Verification items for the finished model (mm, model axes). A direction names the side the tool comes from. Give positions to 0.01 mm unless a question says otherwise; leave off trailing zeros. Order: outer loops, then holes, each group sorted by start corner. A loop starts at its lowest first (then second) coordinate and runs counter-clockwise, first axis right, second up. Notation, with made-up numbers: (57.5, 9) -> (71.5, 9) arc R17 ccw to (71.5, 15) -> close; hole circle Ø3 at (10, -10). An arc over 180 degrees is marked (long way). Return JSON: item names as keys, results as strings. Group by question number.
(1) Cross-section at C-C on x = -0.5. Enter the section's corners in (y, z).
(2) Tool access check on faces 1 (the face through (13.646, 13.93, 0.592)), 2 (the face through (-18.697, -18.759, 3.566)), 3 (the face through (19.359, 19.297, 3.972)). Record the directions out of +Z, -Z, +X, -X, +Y, -Y that give a thin tool (end or side, any length) a straight path to the whole face; none if there is none.
(3) Cross-section at D-D on x = -12.5. Enter the section's corners in (y, z), then the cut area to 3 significant figures.
(4) Release check for a two-part mould opening along X. For faces 4 (the face through (-19.297, 19.359, 3.972)), 5 (the face through (1, -13, 1)), 6 (the face through (20.5, 0, 4)) record: pulls with the +X half, pulls with the -X half, needs draft (parallel to the pull), parting line crosses it, or undercut.
(5) Thickness scan on line 1 along Y through (x, z) = (14, 2.5); line 2 along X through (y, z) = (8, 5); line 3 along Z through (x, y) = (11.5, 3). Record the ranges inside material, lowest first.
(6) Cross-section at A-A on z = 4. Enter the section's corners in (x, y), then the cut area to 4 significant figures.
(7) Cross-section at B-B on y = -13. Enter the section's corners in (x, z).
(8) Depth check by flat-ended pin: pin 1 Ø3 at (x, y) = (12.5, 3) entering from +Z; pin 2 Ø1 at (x, z) = (-8.5, 0.5) entering from +Y; pin 3 Ø1.3 at (y, z) = (-9, 0.5) entering from -X; pin 4 Ø3 at (x, y) = (15.9, 15.9) entering from -Z. Enter the tip coordinate at first touch or a pass-through.
from build123d import *

# Parameters (mm, degrees)
F0_R         = 1.75
F1_DEPTH     = 1.2
F2_DEPTH     = 6
F4_DEPTH     = 10
F5_T1_DEPTH  = 33
F5_T3_DEPTH  = 33
F5_T6_ANGLE  = 90
F5_T8_ANGLE  = 90
F5_T10_ANGLE = 90
F5_T12_ANGLE = 90
F6_DEPTH     = 0.1
F7_DEPTH     = 0.1
F8_DEPTH     = 0.1


# Not quite as in the source:
# - a fillet or chamfer that OpenCascade refuses, or shapes differently, is made with other operations: its cross-section is extruded or revolved along the edge and cut away or added


with BuildPart() as f1:
    # F0 (on Top) → F1 (new body)
    with BuildSketch(Plane.XY):
        with BuildLine():
            Line((-15.9, -19.9), (15.9, -19.9))
            ThreePointArc((15.9, -19.9), (18.7284271247, -18.7284271247), (19.9, -15.9))
            Line((19.9, -15.9), (19.9, 15.9))
            ThreePointArc((19.9, 15.9), (18.7284271247, 18.7284271247), (15.9, 19.9))
            Line((15.9, 19.9), (-15.9, 19.9))
            ThreePointArc((-15.9, 19.9), (-18.7284271247, 18.7284271247), (-19.9, 15.9))
            Line((-19.9, 15.9), (-19.9, -15.9))
            ThreePointArc((-19.9, -15.9), (-18.7284271247, -18.7284271247), (-15.9, -19.9))
        make_face()
        with Locations((-15.9, -15.9)):
            Circle(F0_R, mode=Mode.SUBTRACT)
        with Locations((15.9, -15.9)):
            Circle(F0_R, mode=Mode.SUBTRACT)
        with Locations((-15.9, 15.9)):
            Circle(F0_R, mode=Mode.SUBTRACT)
        with Locations((15.9, 15.9)):
            Circle(F0_R, mode=Mode.SUBTRACT)
    extrude(amount=F1_DEPTH)

    # F0 (on Top) → F2 (join)
    with BuildSketch(Plane.XY):
        with BuildLine():
            Line((-16.5, -20.5), (16.5, -20.5))
            ThreePointArc((16.5, -20.5), (19.3284271247, -19.3284271247), (20.5, -16.5))
            Line((20.5, -16.5), (20.5, 16.5))
            ThreePointArc((20.5, 16.5), (19.3284271247, 19.3284271247), (16.5, 20.5))
            Line((16.5, 20.5), (-16.5, 20.5))
            ThreePointArc((-16.5, 20.5), (-19.3284271247, 19.3284271247), (-20.5, 16.5))
            Line((-20.5, 16.5), (-20.5, -16.5))
            ThreePointArc((-20.5, -16.5), (-19.3284271247, -19.3284271247), (-16.5, -20.5))
        make_face()
        with BuildLine():
            ThreePointArc((19.9, -15.9), (18.7284271247, -18.7284271247), (15.9, -19.9))
            Line((15.9, -19.9), (-15.9, -19.9))
            ThreePointArc((-15.9, -19.9), (-18.7284271247, -18.7284271247), (-19.9, -15.9))
            Line((-19.9, -15.9), (-19.9, 15.9))
            ThreePointArc((-19.9, 15.9), (-18.7284271247, 18.7284271247), (-15.9, 19.9))
            Line((-15.9, 19.9), (15.9, 19.9))
            ThreePointArc((15.9, 19.9), (18.7284271247, 18.7284271247), (19.9, 15.9))
            Line((19.9, 15.9), (19.9, -15.9))
        make_face(mode=Mode.SUBTRACT)
    extrude(amount=F2_DEPTH)

    # F3 (on face) → F4 (cut)
    with BuildSketch(Plane(origin=(0, 0, 0), x_dir=(1, 0, 0), z_dir=(0, 0, -1))):
        with BuildLine():
            ThreePointArc((1, 2.8284271247), (2.1213203436, 2.1213203436), (2.8284271247, 1))
            Line((2.8284271247, 1), (5.9160797831, 1))
            ThreePointArc((5.9160797831, 1), (4.2426406871, 4.2426406871), (1, 5.9160797831))
            Line((1, 5.9160797831), (1, 2.8284271247))
        make_face()
        with BuildLine():
            Line((5.9160797831, -1), (2.8284271247, -1))
            ThreePointArc((2.8284271247, -1), (2.1213203436, -2.1213203436), (1, -2.8284271247))
            Line((1, -2.8284271247), (1, -5.9160797831))
            ThreePointArc((1, -5.9160797831), (4.2426406871, -4.2426406871), (5.9160797831, -1))
        make_face()
        with BuildLine():
            ThreePointArc((-2.8284271247, 1), (-2.1213203436, 2.1213203436), (-1, 2.8284271247))
            Line((-1, 2.8284271247), (-1, 5.9160797831))
            ThreePointArc((-1, 5.9160797831), (-4.2426406871, 4.2426406871), (-5.9160797831, 1))
            Line((-5.9160797831, 1), (-2.8284271247, 1))
        make_face()
        with BuildLine():
            ThreePointArc((1, 7.4330343737), (5.3033008589, 5.3033008589), (7.4330343737, 1))
            Line((7.4330343737, 1), (10.4522724802, 1))
            ThreePointArc((10.4522724802, 1), (7.4246212025, 7.4246212025), (1, 10.4522724802))
            Line((1, 10.4522724802), (1, 7.4330343737))
        make_face()
        with BuildLine():
            Line((-1, -5.9160797831), (-1, -2.8284271247))
            ThreePointArc((-1, -2.8284271247), (-2.1213203436, -2.1213203436), (-2.8284271247, -1))
            Line((-2.8284271247, -1), (-5.9160797831, -1))
            ThreePointArc((-5.9160797831, -1), (-4.2426406871, -4.2426406871), (-1, -5.9160797831))
        make_face()
        with BuildLine():
            Line((10.4522724802, -1), (7.4330343737, -1))
            ThreePointArc((7.4330343737, -1), (5.3033008589, -5.3033008589), (1, -7.4330343737))
            Line((1, -7.4330343737), (1, -10.4522724802))
            ThreePointArc((1, -10.4522724802), (7.4246212025, -7.4246212025), (10.4522724802, -1))
        make_face()
        with BuildLine():
            ThreePointArc((-7.4330343737, 1), (-5.3033008589, 5.3033008589), (-1, 7.4330343737))
            Line((-1, 7.4330343737), (-1, 10.4522724802))
            ThreePointArc((-1, 10.4522724802), (-7.4246212025, 7.4246212025), (-10.4522724802, 1))
            Line((-10.4522724802, 1), (-7.4330343737, 1))
        make_face()
        with BuildLine():
            ThreePointArc((1, 11.9582607431), (8.4852813742, 8.4852813742), (11.9582607431, 1))
            Line((11.9582607431, 1), (14.9666295471, 1))
            ThreePointArc((14.9666295471, 1), (10.6066017178, 10.6066017178), (1, 14.9666295471))
            Line((1, 14.9666295471), (1, 11.9582607431))
        make_face()
        with BuildLine():
            Line((-1, -10.4522724802), (-1, -7.4330343737))
            ThreePointArc((-1, -7.4330343737), (-5.3033008589, -5.3033008589), (-7.4330343737, -1))
            Line((-7.4330343737, -1), (-10.4522724802, -1))
            ThreePointArc((-10.4522724802, -1), (-7.4246212025, -7.4246212025), (-1, -10.4522724802))
        make_face()
        with BuildLine():
            Line((14.9666295471, -1), (11.9582607431, -1))
            ThreePointArc((11.9582607431, -1), (8.4852813742, -8.4852813742), (1, -11.9582607431))
            Line((1, -11.9582607431), (1, -14.9666295471))
            ThreePointArc((1, -14.9666295471), (10.6066017178, -10.6066017178), (14.9666295471, -1))
        make_face()
        with BuildLine():
            ThreePointArc((-11.9582607431, 1), (-8.4852813742, 8.4852813742), (-1, 11.9582607431))
            Line((-1, 11.9582607431), (-1, 14.9666295471))
            ThreePointArc((-1, 14.9666295471), (-10.6066017178, 10.6066017178), (-14.9666295471, 1))
            Line((-14.9666295471, 1), (-11.9582607431, 1))
        make_face()
        with BuildLine():
            ThreePointArc((1, 16.469669092), (11.6672618896, 11.6672618896), (16.469669092, 1))
            Line((16.469669092, 1), (19.4743420942, 1))
            ThreePointArc((19.4743420942, 1), (13.7885822331, 13.7885822331), (1, 19.4743420942))
            Line((1, 19.4743420942), (1, 16.469669092))
        make_face()
        with BuildLine():
            Line((-1, -14.9666295471), (-1, -11.9582607431))
            ThreePointArc((-1, -11.9582607431), (-8.4852813742, -8.4852813742), (-11.9582607431, -1))
            Line((-11.9582607431, -1), (-14.9666295471, -1))
            ThreePointArc((-14.9666295471, -1), (-10.6066017178, -10.6066017178), (-1, -14.9666295471))
        make_face()
        with BuildLine():
            Line((19.4743420942, -1), (16.469669092, -1))
            ThreePointArc((16.469669092, -1), (11.6672618896, -11.6672618896), (1, -16.469669092))
            Line((1, -16.469669092), (1, -19.4743420942))
            ThreePointArc((1, -19.4743420942), (13.7885822331, -13.7885822331), (19.4743420942, -1))
        make_face()
        with BuildLine():
            ThreePointArc((-16.469669092, 1), (-11.6672618896, 11.6672618896), (-1, 16.469669092))
            Line((-1, 16.469669092), (-1, 19.4743420942))
            ThreePointArc((-1, 19.4743420942), (-13.7885822331, 13.7885822331), (-19.4743420942, 1))
            Line((-19.4743420942, 1), (-16.469669092, 1))
        make_face()
        with BuildLine():
            Line((-1, -19.4743420942), (-1, -16.469669092))
            ThreePointArc((-1, -16.469669092), (-11.6672618896, -11.6672618896), (-16.469669092, -1))
            Line((-16.469669092, -1), (-19.4743420942, -1))
            ThreePointArc((-19.4743420942, -1), (-13.7885822331, -13.7885822331), (-1, -19.4743420942))
        make_face()
    extrude(amount=-F4_DEPTH, mode=Mode.SUBTRACT)

    # F5: fillet of radius 2 on 8 edges, made by hand

    # F5_s2 → F5_t1 (cut)
    with BuildSketch(Plane.YZ.offset(-16.5)):
        with BuildLine():
            ThreePointArc((-18.5, 0), (-19.9142135624, 0.5857864376), (-20.5, 2))
            Line((-20.5, 2), (-20.5, 0))
            Line((-20.5, 0), (-18.5, 0))
        make_face()
        with BuildLine():
            ThreePointArc((18.5, 0), (19.9142135624, 0.5857864376), (20.5, 2))
            Line((20.5, 2), (20.5, 0))
            Line((20.5, 0), (18.5, 0))
        make_face()
    extrude(amount=F5_T1_DEPTH, mode=Mode.SUBTRACT)

    # F5_s4 → F5_t3 (cut)
    with BuildSketch(Plane.XZ.offset(-16.5)):
        with BuildLine():
            ThreePointArc((-18.5, 0), (-19.9142135624, 0.5857864376), (-20.5, 2))
            Line((-20.5, 2), (-20.5, 0))
            Line((-20.5, 0), (-18.5, 0))
        make_face()
        with BuildLine():
            ThreePointArc((18.5, 0), (19.9142135624, 0.5857864376), (20.5, 2))
            Line((20.5, 2), (20.5, 0))
            Line((20.5, 0), (18.5, 0))
        make_face()
    extrude(amount=F5_T3_DEPTH, mode=Mode.SUBTRACT)

    # F5_s5 → F5_t6 (revolve, cut)
    with BuildSketch(Plane.XZ.offset(16.5)):
        with BuildLine():
            ThreePointArc((-18.5, 0), (-19.9142135624, 0.5857864376), (-20.5, 2))
            Line((-20.5, 2), (-20.5, 0))
            Line((-20.5, 0), (-18.5, 0))
        make_face()
    revolve(axis=Axis((-16.5, -16.5, 0), (0, 0, 1)), revolution_arc=F5_T6_ANGLE, mode=Mode.SUBTRACT)

    # F5_s7 → F5_t8 (revolve, cut)
    with BuildSketch(Plane.YZ.offset(16.5)):
        with BuildLine():
            ThreePointArc((-18.5, 0), (-19.9142135624, 0.5857864376), (-20.5, 2))
            Line((-20.5, 2), (-20.5, 0))
            Line((-20.5, 0), (-18.5, 0))
        make_face()
    revolve(axis=Axis((16.5, -16.5, 0), (0, 0, 1)), revolution_arc=F5_T8_ANGLE, mode=Mode.SUBTRACT)

    # F5_s9 → F5_t10 (revolve, cut)
    with BuildSketch(Plane.XZ.offset(-16.5)):
        with BuildLine():
            ThreePointArc((18.5, 0), (19.9142135624, 0.5857864376), (20.5, 2))
            Line((20.5, 2), (20.5, 0))
            Line((20.5, 0), (18.5, 0))
        make_face()
    revolve(axis=Axis((16.5, 16.5, 0), (0, 0, 1)), revolution_arc=F5_T10_ANGLE, mode=Mode.SUBTRACT)

    # F5_s11 → F5_t12 (revolve, cut)
    with BuildSketch(Plane.YZ.offset(-16.5)):
        with BuildLine():
            ThreePointArc((18.5, 0), (19.9142135624, 0.5857864376), (20.5, 2))
            Line((20.5, 2), (20.5, 0))
            Line((20.5, 0), (18.5, 0))
        make_face()
    revolve(axis=Axis((-16.5, 16.5, 0), (0, 0, 1)), revolution_arc=F5_T12_ANGLE, mode=Mode.SUBTRACT)

    # F6 (add): a face of the model
    f6_faces = [f1.faces().sort_by_distance(p)[0] for p in [
        (19.9, 0, 3.6),
    ]]
    extrude(f6_faces, amount=F6_DEPTH)

    # F7 (add): a face of the model
    f7_faces = [f1.faces().sort_by_distance(p)[0] for p in [
        (-19.9, 0, 3.6),
    ]]
    extrude(f7_faces, amount=F7_DEPTH)

    # F8 (add): a face of the model
    f8_faces = [f1.faces().sort_by_distance(p)[0] for p in [
        (0, 19.9, 3.6),
    ]]
    extrude(f8_faces, amount=F8_DEPTH)


solid = f1.part
Verdict:
{
 "1": {"outline": "(-20.5, 2) arc R2 ccw to (-18.5, 0) -> (18.5, 0) arc R2 ccw to (20.5, 2) -> (20.5, 6) -> (19.8, 6) -> (19.8, 1.2) -> (-19.9, 1.2) -> (-19.9, 6) -> (-20.5, 6) -> close"},
 "2": {"face 1": "+Z, -Z", "face 2": "+Z", "face 3": "+Z, -Z, +X, +Y"},
 "3": {"outline": "(-20.5, 2) arc R2 ccw to (-18.5, 0) -> (-14.97, 0) -> (-14.97, 1.2) -> (-19.9, 1.2) -> (-19.9, 6) -> (-20.5, 6) -> close; (-10.77, 0) -> (-8.29, 0) -> (-8.29, 1.2) -> (-10.77, 1.2) -> close; (-1, 0) -> (1, 0) -> (1, 1.2) -> (-1, 1.2) -> close; (8.29, 0) -> (10.77, 0) -> (10.77, 1.2) -> (8.29, 1.2) -> close; (14.97, 0) -> (18.5, 0) arc R2 ccw to (20.5, 2) -> (20.5, 6) -> (19.8, 6) -> (19.8, 1.2) -> (14.97, 1.2) -> close", "area": "26.2 mm²"},
 "4": {"face 4": "pulls with the -X half", "face 5": "undercut", "face 6": "pulls with the +X half"},
 "5": {"line 1": "-20.5 to -19.9, 19.8 to 20.5", "line 2": "-20.5 to -19.8, 19.8 to 20.5", "line 3": "0 to 1.2"},
 "6": {"outline": "(-20.5, -16.5) arc R4 ccw to (-16.5, -20.5) -> (16.5, -20.5) arc R4 ccw to (20.5, -16.5) -> (20.5, 16.5) arc R4 ccw to (16.5, 20.5) -> (-16.5, 20.5) arc R4 ccw to (-20.5, 16.5) -> close; hole (-19.9, -15.9) arc R4 ccw to (-15.9, -19.9) -> (15.9, -19.9) arc R4 ccw to (19.9, -15.9) -> (19.8, -15.9) -> (19.8, 15.9) -> (19.9, 15.9) arc R4 ccw to (15.9, 19.9) -> (15.9, 19.8) -> (-15.9, 19.8) -> (-15.9, 19.9) arc R4 ccw to (-19.9, 15.9) -> (-19.8, 15.9) -> (-19.8, -15.9) -> close", "area": "106.5 mm²"},
 "7": {"outline": "(-20.5, 2) arc R2 ccw to (-18.5, 0) -> (-14.53, 0) -> (-14.53, 1.2) -> (-19.8, 1.2) -> (-19.8, 6) -> (-20.5, 6) -> close; (-10.16, 0) -> (-7.48, 0) -> (-7.48, 1.2) -> (-10.16, 1.2) -> close; (-1, 0) -> (1, 0) -> (1, 1.2) -> (-1, 1.2) -> close; (7.48, 0) -> (10.16, 0) -> (10.16, 1.2) -> (7.48, 1.2) -> close; (14.53, 0) -> (18.5, 0) arc R2 ccw to (20.5, 2) -> (20.5, 6) -> (19.8, 6) -> (19.8, 1.2) -> (14.53, 1.2) -> close"},
 "8": {"pin 1": "z = 1.2", "pin 2": "y = 20.23", "pin 3": "x = -20.31", "pin 4": "through"}
}
